The model under review builds one solid part; all positions refer to its coordinate system, in mm. A direction names the side the tool comes from. Coordinates: 2 decimals unless noted, no trailing zeros. Write each loop counter-clockwise with the first axis right and the second up, starting at its lowest first coordinate (ties: lowest second). Pieces come first, ordered by that corner, then holes.
1) Add section C-C, the plane y = 5.5. State the section outline as (x, z) points (3 decimals), then the cut area to 3 significant figures.
2) For line 1 (X direction, y = 2, z = -0.5); line 2 (Z direction, x = 1, y = 1); line 3 (Y direction, x = 2, z = -1.1), list the stretches that pass through material, from the lowest coordinate up.
3) Mouldability with a two-part tool opening along Z and no side actions: class faces 4 (the cylindrical face through (-3.067, 3.219, 2.285)), 5 (the cylindrical face through (-0.966, 9.167, -1.26)), 6 (the flat face through (2, 2, -0.762)) as released by +Z, released by -Z, zero draft, split by the parting line, or undercut.
4) For P1, Ø4, axis at x = -1.5, y = 9.5, coming from the -Z side; P2, Ø1.5, axis at y = 8.5, z = 1, coming from the -X side; P3, Ø2, axis at x = 0, y = 7.5, coming from the +Z side, all flat-tipped, find the tip position at first contact; note any pin that passes through.
5) Machinability: for faces 1 (the flat face through (-2, 6.35, -1)), 2 (the flat face through (2, 2, 0.762)), 3 (the flat face through (0, 12.7, 0)), which of the approach directions +Z, -Z, +X, -X, +Y, -Y give a long, thin tool a straight path to every point of the face, cutting with its end or side? Answer none if there is none.
6) Add section A-A, the plane y = 2.5. State the section outline as (x, z) points (3 decimals), then the cut area to 3 significant figures.
from build123d import *

# Parameters (mm, degrees)
SKETCH1_W           = 6.858
SKETCH1_H           = 5.334
BOSS_EXTRUDE1_DEPTH = 6.35
SKETCH4_W           = 1.397
SKETCH4_H           = 1.524
SKETCH4_W_2         = 1.524
SKETCH4_H_2         = 1.397
CUT_EXTRUDE1_DEPTH  = 3.556
SKETCH5_W           = 1.524
SKETCH5_H           = 1.143
BOSS_EXTRUDE4_DEPTH = 0.254
FILLET1_R           = 0.127
FILLET3_R           = 0.635
FILLET4_R           = 0.254
FILLET5_R           = 0.254
FILLET6_R           = 1.27
SKETCH6_R           = 1.5875
BOSS_EXTRUDE5_DEPTH = 6.35
FILLET8_R           = 0.635


with BuildPart() as part:
    # Sketch1 → Boss-Extrude1 (new body)
    with BuildSketch(Plane(origin=(0, 0, 0), x_dir=(1, 0, 0), z_dir=(0, 1, 0))):
        Rectangle(SKETCH1_W, SKETCH1_H)
    extrude(amount=BOSS_EXTRUDE1_DEPTH)

    # Sketch4 → Cut-Extrude1 (cut)
    with BuildSketch(Plane.XZ):
        with Locations((-1.4605, 0)):
            Rectangle(SKETCH4_W, SKETCH4_H)
        Rectangle(SKETCH4_W_2, SKETCH4_H)
        with Locations((1.4605, 0)):
            Rectangle(SKETCH4_W, SKETCH4_H)
        with Locations((0, -1.4605)):
            Rectangle(SKETCH4_W_2, SKETCH4_H_2)
        with Locations((0, 1.4605)):
            Rectangle(SKETCH4_W_2, SKETCH4_H_2)
    extrude(amount=-CUT_EXTRUDE1_DEPTH, mode=Mode.SUBTRACT)

    # Sketch5 → Boss-Extrude4 (add)
    with BuildSketch(Plane(origin=(0, 0, 2.159), x_dir=(-1, 0, 0), z_dir=(0, 0, -1))):
        with Locations((0, 2.3495)):
            Rectangle(SKETCH5_W, SKETCH5_H)
    extrude(amount=BOSS_EXTRUDE4_DEPTH)

    # Fillet1
    fillet1_edges = [part.edges().sort_by_distance(p)[0] for p in [
        (0, 1.778, 1.905),
        (0, 2.921, 1.905),
    ]]
    fillet(fillet1_edges, radius=FILLET1_R)

    # Fillet3
    fillet3_edges = [part.edges().sort_by_distance(p)[0] for p in [
        (3.429, 3.175, 2.667),
        (-3.429, 3.175, -2.667),
        (3.429, 3.175, -2.667),
    ]]
    fillet(fillet3_edges, radius=FILLET3_R)

    # Fillet4
    fillet4_edges = [part.edges().sort_by_distance(p)[0] for p in [
        (-1.4605, 0, -0.762),
        (-2.159, 0, 0),
        (0.762, 0, 1.4605),
        (1.4605, 0, -0.762),
        (0.762, 0, -1.4605),
        (0, 0, -2.159),
        (-0.762, 0, -1.4605),
        (2.159, 0, 0),
        (1.4605, 0, 0.762),
        (0, 0, 2.159),
        (-0.762, 0, 1.4605),
        (-1.4605, 0, 0.762),
    ]]
    fillet(fillet4_edges, radius=FILLET4_R)

    # Fillet5
    # the kernel refuses this fillet: 0.254 mm, written as the material it takes off along each edge
    with BuildSketch(Plane(origin=(1.016, 0.254, -1.016), x_dir=(0, 0, 1), z_dir=(-1, 0, 0))) as fillet5_piece_1_section:
        Polygon((0, 0), (FILLET5_R, 0), (FILLET5_R, -FILLET5_R), (0, -FILLET5_R), align=None)
    fillet5_piece_1 = extrude(amount=FILLET5_R, mode=Mode.PRIVATE)
    fillet5_piece_1 = fillet5_piece_1 - Plane(origin=(1.016, 0.254, -1.016), x_dir=(0, 0.7071067811865475, -0.7071067811865475), z_dir=(-1, 0, 0)) * Sphere(FILLET5_R, mode=Mode.PRIVATE)
    add(fillet5_piece_1, mode=Mode.SUBTRACT)
    with BuildSketch(Plane(origin=(1.016, 0.254, 1.016), x_dir=(0, 0, -1), z_dir=(-1, 0, 0))) as fillet5_piece_2_section:
        Polygon((0, 0), (FILLET5_R, 0), (FILLET5_R, FILLET5_R), (0, FILLET5_R), align=None)
    fillet5_piece_2 = extrude(amount=FILLET5_R, mode=Mode.PRIVATE)
    fillet5_piece_2 = fillet5_piece_2 - Plane(origin=(1.016, 0.254, 1.016), x_dir=(0, 0.7071067811865475, 0.7071067811865475), z_dir=(-1, 0, 0)) * Sphere(FILLET5_R, mode=Mode.PRIVATE)
    add(fillet5_piece_2, mode=Mode.SUBTRACT)
    with BuildSketch(Plane(origin=(-1.016, 0.254, -1.016), x_dir=(1, 0, 0), z_dir=(0, 0, 1))) as fillet5_piece_3_section:
        Polygon((0, 0), (FILLET5_R, 0), (FILLET5_R, -FILLET5_R), (0, -FILLET5_R), align=None)
    fillet5_piece_3 = extrude(amount=FILLET5_R, mode=Mode.PRIVATE)
    fillet5_piece_3 = fillet5_piece_3 - Plane(origin=(-1.016, 0.254, -1.016), x_dir=(-0.7071067811865475, 0.7071067811865475, 0), z_dir=(0, 0, 1)) * Sphere(FILLET5_R, mode=Mode.PRIVATE)
    add(fillet5_piece_3, mode=Mode.SUBTRACT)
    with BuildSketch(Plane(origin=(-1.016, 0.254, 1.016), x_dir=(1, 0, 0), z_dir=(0, 0, -1))) as fillet5_piece_4_section:
        Polygon((0, 0), (FILLET5_R, 0), (FILLET5_R, FILLET5_R), (0, FILLET5_R), align=None)
    fillet5_piece_4 = extrude(amount=FILLET5_R, mode=Mode.PRIVATE)
    fillet5_piece_4 = fillet5_piece_4 - Plane(origin=(-1.016, 0.254, 1.016), x_dir=(-0.7071067811865475, 0.7071067811865475, 0), z_dir=(0, 0, -1)) * Sphere(FILLET5_R, mode=Mode.PRIVATE)
    add(fillet5_piece_4, mode=Mode.SUBTRACT)
    with BuildSketch(Plane(origin=(-0.762, 0.254, -0.762), x_dir=(-1, 0, 0), z_dir=(0, 1, 0)), Plane(origin=(0.762, 0.254, -0.762), x_dir=(0, 0, -1), z_dir=(0, 1, 0))) as fillet5_piece_5:
        with BuildLine():
            CenterArc((FILLET5_R, -FILLET5_R), FILLET5_R, 90, 90)
            Line((0, -FILLET5_R), (0, 0))
            Line((0, 0), (FILLET5_R, 0))
        make_face()
    extrude(amount=3.302, mode=Mode.SUBTRACT)
    with BuildSketch(Plane(origin=(-0.762, 0.254, 0.762), x_dir=(-1, 0, 0), z_dir=(0, 1, 0)), Plane(origin=(0.762, 0.254, 0.762), x_dir=(0, 0, 1), z_dir=(0, 1, 0))) as fillet5_piece_6:
        with BuildLine():
            CenterArc((FILLET5_R, FILLET5_R), FILLET5_R, 180, 90)
            Line((0, FILLET5_R), (0, 0))
            Line((0, 0), (FILLET5_R, 0))
        make_face()
    extrude(amount=3.302, mode=Mode.SUBTRACT)

    # Fillet6
    fillet6_edges = [part.edges().sort_by_distance(p)[0] for p in [
        (-3.429, 3.175, 2.667),
    ]]
    fillet(fillet6_edges, radius=FILLET6_R)

    # Sketch6 → Boss-Extrude5 (add)
    with BuildSketch(Plane(origin=(0, 6.35, 0), x_dir=(1, 0, 0), z_dir=(0, 1, 0))):
        with Locations(Location((0, 0, 0), (0, 0, 270))):
            Circle(SKETCH6_R)
    extrude(amount=BOSS_EXTRUDE5_DEPTH)

    # Fillet8
    fillet8_edges = [part.edges().sort_by_distance(p)[0] for p in [
        (0, 12.7, -1.5875),
    ]]
    fillet(fillet8_edges, radius=FILLET8_R)


solid = part.part
Geometry results:
1. outline: (-3.429, -2.032) arc R0.635 ccw to (-2.794, -2.667) - (2.794, -2.667) arc R0.635 ccw to (3.429, -2.032) - (3.429, 2.032) arc R0.635 ccw to (2.794, 2.667) - (-2.159, 2.667) arc R1.27 ccw to (-3.429, 1.397) - close
1. area: 36.0 mm2
2. line 1: x = -3.43 to -2.16, 2.16 to 3.43
2. line 2: z = -2.67 to -0.76, 0.76 to 2.67
2. line 3: y = 0 to 6.35
3. face 4: released by +Z
3. face 5: split by the parting line
3. face 6: undercut
4. P1: stops at z = -1.59
4. P2: stops at x = -1.57
4. P3: stops at z = 1.59
5. face 1: +Y
5. face 2: -Y
5. face 3: +Z, -Z, +X, -X, +Y
6. outline: (-3.429, -2.032) arc R0.635 ccw to (-2.794, -2.667) - (2.794, -2.667) arc R0.635 ccw to (3.429, -2.032) - (3.429, 2.032) arc R0.635 ccw to (2.794, 2.667) - (-2.159, 2.667) arc R1.27 ccw to (-3.429, 1.397) - close; hole (-2.159, -0.762) - (-1.016, -0.762) arc R0.254 cw to (-0.762, -1.016) - (-0.762, -2.159) - (0.762, -2.159) - (0.762, -1.016) arc R0.254 cw to (1.016, -0.762) - (2.159, -0.762) - (2.159, 0.762) - (1.016, 0.762) arc R0.254 cw to (0.762, 1.016) - (0.762, 1.905) - (-0.762, 1.905) - (-0.762, 1.016) arc R0.254 cw to (-1.016, 0.762) - (-2.159, 0.762) - close
6. area: 25.5 mm2
